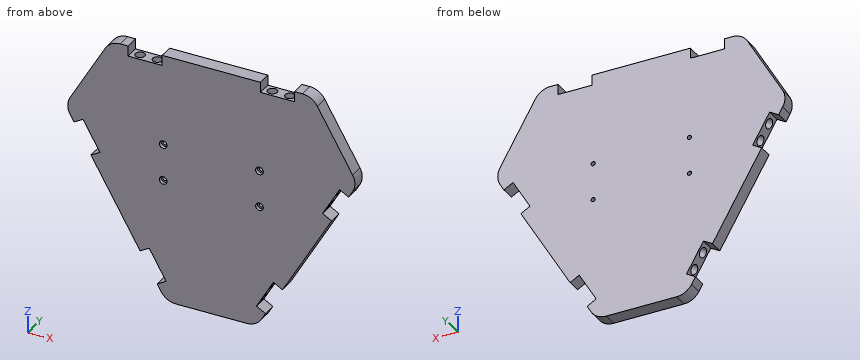
from build123d import *

# Parameters (mm, degrees)
BOSS_EXTRUDE1_DEPTH            = 4
CHAMFER1_SIZE                  = 52
SKETCH4_W                      = 19.5
SKETCH4_H                      = 8
SKETCH4_R                      = 2
CUT_EXTRUDE1_DEPTH             = 6
SKETCH4_2_R                    = 2
CUT_EXTRUDE2_DEPTH             = 16
SKETCH9_R                      = 2.75
CUT_EXTRUDE3_DEPTH             = 7
CRVPATTERN1_START              = -63.508529611
CRVPATTERN1_OUTLINE_W          = 19.5
CRVPATTERN1_OUTLINE_H          = 8
CRVPATTERN1_DEPTH              = 6
CRVPATTERN1_START_2            = -57.508529611
CRVPATTERN1_2_OUTLINE_R        = 2.75
CRVPATTERN1_2_DEPTH            = 7
CRVPATTERN1_START_3            = -50.508529611
CRVPATTERN1_3_OUTLINE_R        = 2
CRVPATTERN1_3_DEPTH            = 3
CRVPATTERN1_START_4            = 57.508529611
CRVPATTERN1_4_OUTLINE_W        = 19.5
CRVPATTERN1_4_OUTLINE_H        = 8
CRVPATTERN1_4_DEPTH            = 6
CRVPATTERN1_START_5            = 50.508529611
CRVPATTERN1_5_OUTLINE_R        = 2.75
CRVPATTERN1_5_DEPTH            = 7
CRVPATTERN1_START_6            = 47.508529611
CRVPATTERN1_6_OUTLINE_R        = 2
CRVPATTERN1_6_DEPTH            = 3
FILLET1_R                      = 10
CBORE_FOR_M2_SHCS1_D           = 2.4
CBORE_FOR_M2_SHCS1_CBORE_D     = 4.4
CBORE_FOR_M2_SHCS1_CBORE_DEPTH = 2


# Read off the part's stored shape, not the designer's step: CrvPattern1
with BuildPart() as part:
    # Sketch1 → Boss-Extrude1 (new, symmetric)
    with BuildSketch(Plane(origin=(0, 0, 0), x_dir=(1, 0, 0), z_dir=(0, 1, 0))):
        Polygon((110, -63.508529611), (0, 127.017059222), (-110, -63.508529611), align=None)
    extrude(amount=BOSS_EXTRUDE1_DEPTH, both=True)

    # Chamfer1
    chamfer1_edges = [part.edges().sort_by_distance(p)[0] for p in [
        (-110, 0, 63.508529611),
        (0, 0, -127.017059222),
        (110, 0, 63.508529611),
    ]]
    chamfer(chamfer1_edges, length=CHAMFER1_SIZE)

    # Sketch4 → Cut-Extrude1 (cut)
    with BuildSketch(Plane(origin=(4.375288244, 0, 63.508529611), x_dir=(-1, 0, 0), z_dir=(0, 0, -1))):
        with Locations((42.375288244, 0)):
            Rectangle(SKETCH4_W, SKETCH4_H)
        with Locations((37.375288244, 0)):
            Circle(SKETCH4_R, mode=Mode.SUBTRACT)
        with Locations((47.375288244, 0)):
            Circle(SKETCH4_R, mode=Mode.SUBTRACT)
    cut_extrude1 = extrude(amount=CUT_EXTRUDE1_DEPTH, mode=Mode.SUBTRACT)

    # Sketch4<2> → Cut-Extrude2 (cut)
    with BuildSketch(Plane(origin=(4.375288244, 0, 63.508529611), x_dir=(-1, 0, 0), z_dir=(0, 0, -1))):
        with Locations((47.375288244, 0)):
            Circle(SKETCH4_2_R)
        with Locations((37.375288244, 0)):
            Circle(SKETCH4_2_R)
    cut_extrude2 = extrude(amount=CUT_EXTRUDE2_DEPTH, mode=Mode.SUBTRACT)

    # Sketch9 → Cut-Extrude3 (cut)
    with BuildSketch(Plane.XY.offset(57.508529611)):
        with Locations((-43, 0)):
            Circle(SKETCH9_R)
        with Locations((-33, 0)):
            Circle(SKETCH9_R)
    cut_extrude3 = extrude(amount=-CUT_EXTRUDE3_DEPTH, mode=Mode.SUBTRACT)

    # Mirror1: Cut-Extrude1, Cut-Extrude2, Cut-Extrude3 across plane
    add(cut_extrude1.mirror(Plane(origin=(0, 0, 0), x_dir=(0, 0, 1), z_dir=(1, 0, 0))), mode=Mode.SUBTRACT)
    add(cut_extrude2.mirror(Plane(origin=(0, 0, 0), x_dir=(0, 0, 1), z_dir=(1, 0, 0))), mode=Mode.SUBTRACT)
    add(cut_extrude3.mirror(Plane(origin=(0, 0, 0), x_dir=(0, 0, 1), z_dir=(1, 0, 0))), mode=Mode.SUBTRACT)

    # CrvPattern1 outline → CrvPattern1 (cut)
    with BuildSketch(Plane(origin=(0, 0, 0), x_dir=(0.499999999999987, 0, -0.8660254037844463), z_dir=(0.8660254037844461, 0, 0.49999999999998707)).offset(CRVPATTERN1_START)):
        with Locations((-38, 0)):
            Rectangle(CRVPATTERN1_OUTLINE_W, CRVPATTERN1_OUTLINE_H)
        with Locations((38, 0)):
            Rectangle(CRVPATTERN1_OUTLINE_W, CRVPATTERN1_OUTLINE_H)
    extrude(amount=CRVPATTERN1_DEPTH, mode=Mode.SUBTRACT)

    # CrvPattern1 2 outline → CrvPattern1 2 (cut)
    with BuildSketch(Plane(origin=(0, 0, 0), x_dir=(0.499999999999987, 0, -0.8660254037844463), z_dir=(0.8660254037844461, 0, 0.49999999999998707)).offset(CRVPATTERN1_START_2)):
        with Locations((-43, 0)):
            Circle(CRVPATTERN1_2_OUTLINE_R)
        with Locations((-33, 0)):
            Circle(CRVPATTERN1_2_OUTLINE_R)
        with Locations((33, 0)):
            Circle(CRVPATTERN1_2_OUTLINE_R)
        with Locations((43, 0)):
            Circle(CRVPATTERN1_2_OUTLINE_R)
    extrude(amount=CRVPATTERN1_2_DEPTH, mode=Mode.SUBTRACT)

    # CrvPattern1 3 outline → CrvPattern1 3 (cut)
    with BuildSketch(Plane(origin=(0, 0, 0), x_dir=(0.499999999999987, 0, -0.8660254037844463), z_dir=(0.8660254037844461, 0, 0.49999999999998707)).offset(CRVPATTERN1_START_3)):
        with Locations((-43, 0)):
            Circle(CRVPATTERN1_3_OUTLINE_R)
        with Locations((-33, 0)):
            Circle(CRVPATTERN1_3_OUTLINE_R)
        with Locations((33, 0)):
            Circle(CRVPATTERN1_3_OUTLINE_R)
        with Locations((43, 0)):
            Circle(CRVPATTERN1_3_OUTLINE_R)
    extrude(amount=CRVPATTERN1_3_DEPTH, mode=Mode.SUBTRACT)

    # CrvPattern1 4 outline → CrvPattern1 4 (cut)
    with BuildSketch(Plane(origin=(0, 0, 0), x_dir=(0.500000000000001, 0, 0.866025403784438), z_dir=(0.866025403784438, 0, -0.500000000000001)).offset(CRVPATTERN1_START_4)):
        with Locations((-38, 0)):
            Rectangle(CRVPATTERN1_4_OUTLINE_W, CRVPATTERN1_4_OUTLINE_H)
        with Locations((38, 0)):
            Rectangle(CRVPATTERN1_4_OUTLINE_W, CRVPATTERN1_4_OUTLINE_H)
    extrude(amount=CRVPATTERN1_4_DEPTH, mode=Mode.SUBTRACT)

    # CrvPattern1 5 outline → CrvPattern1 5 (cut)
    with BuildSketch(Plane(origin=(0, 0, 0), x_dir=(0.500000000000001, 0, 0.866025403784438), z_dir=(0.866025403784438, 0, -0.500000000000001)).offset(CRVPATTERN1_START_5)):
        with Locations((-43, 0)):
            Circle(CRVPATTERN1_5_OUTLINE_R)
        with Locations((-33, 0)):
            Circle(CRVPATTERN1_5_OUTLINE_R)
        with Locations((33, 0)):
            Circle(CRVPATTERN1_5_OUTLINE_R)
        with Locations((43, 0)):
            Circle(CRVPATTERN1_5_OUTLINE_R)
    extrude(amount=CRVPATTERN1_5_DEPTH, mode=Mode.SUBTRACT)

    # CrvPattern1 6 outline → CrvPattern1 6 (cut)
    with BuildSketch(Plane(origin=(0, 0, 0), x_dir=(0.500000000000001, 0, 0.866025403784438), z_dir=(0.866025403784438, 0, -0.500000000000001)).offset(CRVPATTERN1_START_6)):
        with Locations((-43, 0)):
            Circle(CRVPATTERN1_6_OUTLINE_R)
        with Locations((-33, 0)):
            Circle(CRVPATTERN1_6_OUTLINE_R)
        with Locations((33, 0)):
            Circle(CRVPATTERN1_6_OUTLINE_R)
        with Locations((43, 0)):
            Circle(CRVPATTERN1_6_OUTLINE_R)
    extrude(amount=CRVPATTERN1_6_DEPTH, mode=Mode.SUBTRACT)

    # Fillet1
    fillet1_edges = [part.edges().sort_by_distance(p)[0] for p in [
        (58, 0, 63.508529611),
        (-58, 0, 63.508529611),
        (-26, 0, -81.983738225),
        (-84, 0, 18.475208614),
        (26, 0, -81.983738225),
        (84, 0, 18.475208614),
    ]]
    fillet(fillet1_edges, radius=FILLET1_R)

    # CBORE for M2 SHCS1 (through all)
    with Locations(Plane(origin=(0, -4, 0), x_dir=(-1, 0, 0), z_dir=(0, -1, 0))):
        with Locations((-27.65, -10.65), (27.65, 10.65), (27.65, -10.65), (-27.65, 10.65)):
            CounterBoreHole(CBORE_FOR_M2_SHCS1_D / 2, CBORE_FOR_M2_SHCS1_CBORE_D / 2, CBORE_FOR_M2_SHCS1_CBORE_DEPTH)


solid = part.part
Geometry check sheet. Reference: the model listing, model coordinates, mm. Coordinates: 2 decimals unless noted, no trailing zeros. Order: outer loops, then holes, each group sorted by start corner. A loop starts at its lowest first (then second) coordinate and runs counter-clockwise, first axis right, second up. Notation, with made-up numbers: (60, 19) - (74, 19) arc R15 ccw to (74, 30) - close; hole circle Ø7 at (4.25, 61.25). An arc over 180 degrees is marked (long way). Answer in a Markdown table with one row per item. Add a question column.
1) Material ranges on line 1 along X through (y, z) = (-1, -62); line 2 along Z through (x, y) = (-30, -0.75); line 3 along Y through (x, z) = (33, 54), recorded low to high. Write a range as [from, to].
2) Cross-section at C-C, the plane y = 0. State how many separate pieces and enclosed holes the cut face has, then the cut area to 3 significant figures.
3) Cross-section at D-D, the plane z = -37.5. Record the cut outline in (x, y), then the cut area to 3 significant figures.
4) Gauge pin test, flat ends, axial feed: P1, Ø4.5, axis at x = 33.5, y = -1.5, coming from the +Z side; P2, Ø4.5, axis at x = 43, y = 0, coming from the -Z side; P3, Ø1, axis at y = 0, z = -44.5, coming from the -X side. Record the tip position at first contact, or that the pin passes through.
5) Cross-section at B-B, the plane z = 25.5. Record the cut outline in (x, y).
6) Cross-section at A-A, the plane x = 43. Record the cut outline in (y, z), then the cut area to 3 significant figures.
Check result:
| question | item | result |
|---|---|---|
| 1 | line 1 | x = [-30.61, -26.51], [-19.06, 19.06], [26.51, 30.61] |
| 1 | line 2 | z = [-75.06, -72.46], [-63.06, -58.48], [-52.37, 57.51] |
| 1 | line 3 | y = [-4, -2.75], [2.75, 4] |
| 2 | separate pieces | 1 |
| 2 | enclosed holes | 4 |
| 2 | area | 16,100 mm² |
| 3 | outline | (-51.68, -4) - (51.68, -4) - (51.68, 4) - (-51.68, 4) - close |
| 3 | area | 827 mm² |
| 4 | P1 | stops at z = 57.51 |
| 4 | P2 | stops at z = -56.22 |
| 4 | P3 | stops at x = -47.93 |
| 5 | outline | (-79.94, -4) - (79.94, -4) - (79.94, 4) - (-79.94, 4) - close |
| 6 | outline | (-4, -52.54) - (4, -52.54) - (4, 57.51) - (2.75, 57.51) - (2.75, 50.51) - (2, 50.51) - (2, 47.51) - (-2, 47.51) - (-2, 50.51) - (-2.75, 50.51) - (-2.75, 57.51) - (-4, 57.51) - close |
| 6 | area | 830 mm² |
